CAD build for the part. Positions are in the model's coordinates, mm. A direction names the side the tool comes from. Round coordinates to 2 decimals unless told otherwise and drop trailing zeros. Loops run counter-clockwise (first coordinate to the right, second up) from the corner with the lowest first, then second, coordinate; pieces in that order, holes last. Notation, with made-up numbers: (65.5, 4.25) - (107.5, 4.25) arc R15 ccw to (107.5, 29.25) - close; hole circle Ø4 at (72.25, 78). An arc over 180 degrees is marked (long way). Use one line per item in the form item = value.
from build123d import *

# Parameters (mm, degrees)
F3_START = -5
F2_R     = 37.5
F2_R_2   = 12.5
F3_DEPTH = 10


with BuildPart() as f1:
    # F0 (on Front) → F1 (revolve)
    with BuildSketch(Plane.XZ):
        with BuildLine():
            Line((0, 95), (0, 37.5))
            Line((0, 37.5), (20, 37.5))
            Line((20, 37.5), (20, 95))
            Line((20, 95), (15, 95))
            Line((15, 95), (15, 84))
            ThreePointArc((15, 84), (10, 79), (5, 84))
            Line((5, 84), (5, 95))
            Line((5, 95), (0, 95))
        make_face()
    revolve(axis=Axis((28.1461849809, 0, 0), (1, 0, 0)))

    # F2 (on face) → F3 (join)
    with BuildSketch(Plane.YZ.offset(20).offset(F3_START)):
        Circle(F2_R)
        Circle(F2_R_2, mode=Mode.SUBTRACT)
    extrude(amount=-F3_DEPTH)


solid = f1.part
1) Drill centre lines: probe 1 along Z at (x, y) = (18.9, 0); probe 2 along X at (y, z) = (-68.5, 59). Where is each one in solid material? Low to high.
Report:
probe_1 = -95 to -37.5, 37.5 to 95
probe_2 = 0 to 5, 15 to 20
2) Two-plate mould, pull along Z, no slides. Class faces 1 (the flat face through (15, -9, 9)), 2 (the flat face through (0, -1, 41)), 3 (the flat face through (5, -9, 9)), 4 (the cylindrical face through (2.46, 92.74, -20.59)): +Z half, -Z half, draft (parallel to the pull), parting line (faces both ways), or undercut.
Report:
face_1 = undercut
face_2 = draft
face_3 = undercut
face_4 = parting line
3) Flat gauge pins, fed straight in: pin 1 (10 mm diameter, centred on x = 14.5, y = 66.5, fed in from -Z); pin 2 (2 mm diameter, centred on x = 5.5, y = 37, fed in from -Z); pin 3 (3 mm diameter, centred on y = 11, z = -13.5, fed in from -X). Where does each tip first touch, or does it go through?
Report:
pin_1 = -72.39
pin_2 = -87.86
pin_3 = 5
4) Tool access for faces 5 (the flat face through (5, 84, -7)), 6 (the cylindrical face through (17.54, 14.36, 34.64)), 7 (the flat face through (20, -1, -41)), 8 (the cylindrical face through (17.46, 92.74, -20.59)), 9 (the cylindrical face through (2.54, 14.36, 34.64)): list every direction of +Z, -Z, +X, -X, +Y, -Y with a clear straight run to the whole face (end or side of a thin tool).
Report:
face_5 = none
face_6 = +X
face_7 = +Z, -Z, +X, +Y, -Y
face_8 = +X, -X
face_9 = -X
5) Slice it at A-A (z = 0). Write the cut outline in (x, y), plus the area to 3 significant figures.
Report:
outline = (0, -95) - (5, -95) - (5, -84) arc R5 cw to (15, -84) - (15, -95) - (20, -95) - (20, -37.5) - (15, -37.5) - (15, -12.5) - (5, -12.5) - (5, -37.5) - (0, -37.5) - close; (0, 37.5) - (5, 37.5) - (5, 12.5) - (15, 12.5) - (15, 37.5) - (20, 37.5) - (20, 95) - (15, 95) - (15, 84) arc R5 cw to (5, 84) - (5, 95) - (0, 95) - close
area = 2,500 mm^2
